Job drawing, mm, ordinate dimensions from the low corner. One solid piece. Coordinates: 2 decimals unless noted, no trailing zeros. Write each loop counter-clockwise with the first axis right and the second up, starting at its lowest first coordinate (ties: lowest second). Pieces come first, ordered by that corner, then holes. Notation, with made-up numbers: (16, 28) - (38, 28) arc R27 ccw to (38, 61) - close; hole circle Ø8 at (2, -38). An arc over 180 degrees is marked (long way). Use one line per item in the form item = value. Start each with the question number.
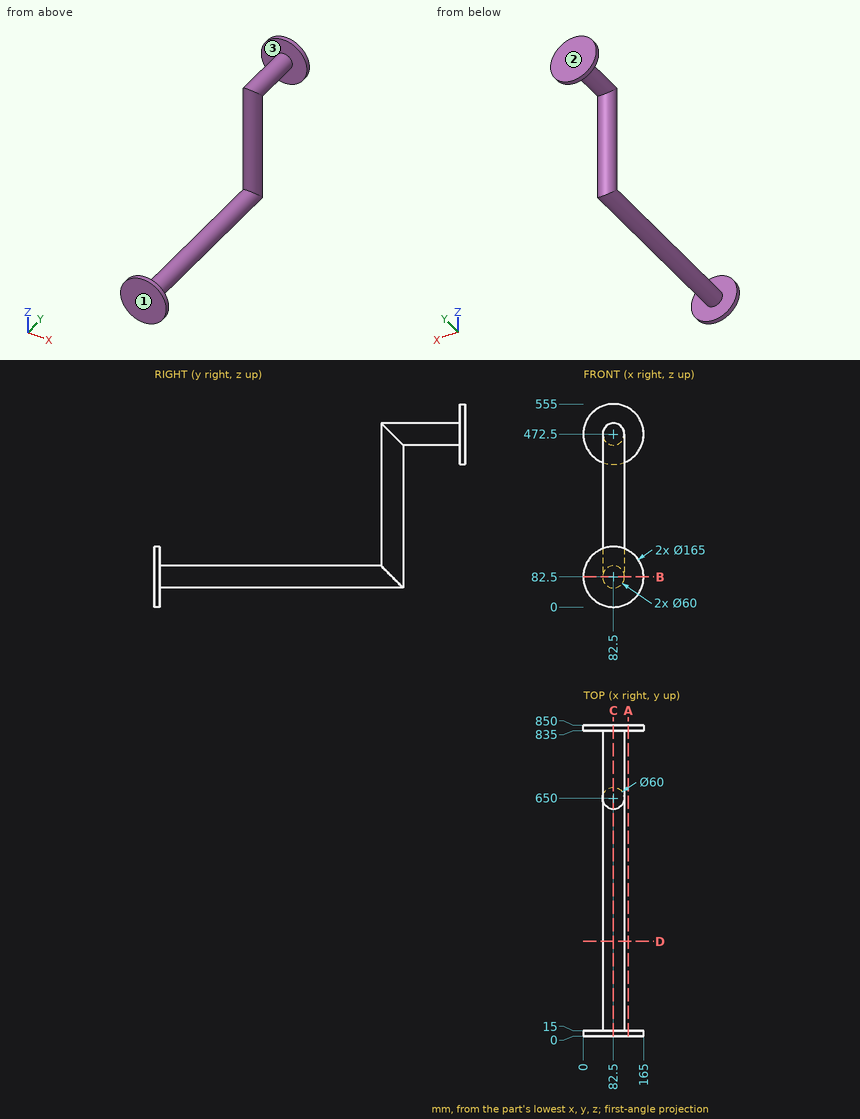
Q1. Drill centre lines: probe 1 along Y at (x, z) = (80, 416); probe 2 along X at (y, z) = (444.5, 80); probe 3 along Y at (x, z) = (86, 224). Where is each one in solid material? Low to high.
Q2. Mould opens along Y. For the marked faces 1, 2 and 3 say: released by +Y, released by -Y, zero draft, split by the parting line, or undercut.
Q3. Slice it at A-A (x = 123.5). List the corners of the cut face in (y, z), plus the area to 3 significant figures.
Q4. Slice it at C-C (x = 82.5). List the corners of the cut face in (y, z), plus the area to 4 significant figures.
Q5. Slice it at D-D (y = 258.5). List the corners of the cut face in (x, z).
Q6. Pin check, flat tips, straight feed: P1, Ø1.5, axis at y = 354.5, z = 88.5, coming from the -X side; P2, Ø8, axis at y = 258.5, z = 101.5, coming from the -X side; P3, Ø3, axis at y = 655.5, z = 107, coming from the -X side. Stop position of each tip, or through.
Q7. Slice it at B-B (z = 82.5). List the corners of the cut face in (x, y).
Solution:
q1.probe_1 = 620.1 to 679.9, 835 to 850
q1.probe_2 = 52.6 to 112.4
q1.probe_3 = 620.2 to 679.8
q2.face_1 = released by -Y
q2.face_2 = released by +Y
q2.face_3 = undercut
q3.outline = (0, 10.91) - (15, 10.91) - (15, 154.09) - (0, 154.09) - close; (835, 400.91) - (850, 400.91) - (850, 544.09) - (835, 544.09) - close
q3.area = 4,300 mm2
q4.outline = (0, 0) - (15, 0) - (15, 52.5) - (680, 52.5) - (680, 442.5) - (835, 442.5) - (835, 390) - (850, 390) - (850, 555) - (835, 555) - (835, 502.5) - (620, 502.5) - (620, 112.5) - (15, 112.5) - (15, 165) - (0, 165) - close
q4.area = 77,550 mm2
q5.outline = circle Ø60 at (82.5, 82.5)
q6.P1 = 52.96
q6.P2 = 56.52
q6.P3 = 52.77
q7.outline = (0, 0) - (165, 0) - (165, 15) - (112.5, 15) - (112.5, 650) arc R30 ccw to (52.5, 650) - (52.5, 15) - (0, 15) - close
